The listing builds one solid part. Answer for the finished solid, in the listing's coordinates (mm). A direction names the side the tool comes from. Give positions to 0.01 mm unless a question says otherwise; leave off trailing zeros. Loops run counter-clockwise (first coordinate to the right, second up) from the corner with the lowest first, then second, coordinate; pieces in that order, holes last. Notation, with made-up numbers: M 44,25.25 L 61,25.25 A17 ccw 61,36.25 Z; hole C -39,60.25 d4. An arc over 180 degrees is marked long. Use one line per item in the form item = value. Start each with the question number.
1. The part is cut by section A-A (z = -1). Write down the section's boundary in (x, y).
2. The part is cut by section C-C (y = 14). Write down the section's boundary in (x, z), and give its area (3 significant figures).
3. Each of these flat-tipped pins is pushed along its axis until it touches: pin 1 Ø12 at (y, z) = (31.5, 9) entering from +X; pin 2 Ø19 at (x, z) = (2, -1) entering from +Y. Where does it stop, or does it pass through?
4. The part is cut by section B-B (x = -1.5). Write down the section's boundary in (y, z), and give its area (3 significant figures).
5. Straight lines are drawn through the part: line 1 (X direction, y = 32, z = -8.5); line 2 (Y direction, x = -4, z = 17). For each, find the intervals that lie inside material, in ascending order. Write a range as from..to.
6. For faces 1 (the face through (-25, 40, 0)), 2 (the face through (-23.75, 21, 0)), determine the directions among +Z, -Z, +X, -X, +Y, -Y from which every point of the face is accessible in a straight line to the end or side of a thin tool.
from build123d import *

# Parameters (mm, degrees)
SKETCH1_W           = 51.5
SKETCH1_H           = 37.5
BOSS_EXTRUDE1_DEPTH = 40
SKETCH2_W           = 49.5
SKETCH2_H           = 38
CUT_EXTRUDE1_DEPTH  = 38.5
FILLET1_R           = 1
FILLET2_R           = 2


with BuildPart() as part:
    # Sketch1 → Boss-Extrude1 (new body)
    with BuildSketch(Plane(origin=(0, 0, 0), x_dir=(1, 0, 0), z_dir=(0, 1, 0))):
        Rectangle(SKETCH1_W, SKETCH1_H)
    extrude(amount=BOSS_EXTRUDE1_DEPTH)

    # Sketch2 → Cut-Extrude1 (cut, through all)
    with BuildSketch(Plane.XY.offset(18.75)):
        with Locations((1, 21)):
            Rectangle(SKETCH2_W, SKETCH2_H)
    extrude(amount=-CUT_EXTRUDE1_DEPTH, mode=Mode.SUBTRACT)

    # Fillet1
    fillet1_edges = [part.edges().sort_by_distance(p)[0] for p in [
        (-23.75, 2, 0),
    ]]
    fillet(fillet1_edges, radius=FILLET1_R)

    # Fillet2
    fillet2_edges = [part.edges().sort_by_distance(p)[0] for p in [
        (-25.75, 0, 0),
    ]]
    fillet(fillet2_edges, radius=FILLET2_R)


solid = part.part
Derived:
q1.outline = M -25.75,2 A2 ccw -23.75,0 L 25.75,0 L 25.75,2 L -22.75,2 A1 cw -23.75,3 L -23.75,40 L -25.75,40 Z
q2.outline = M -25.75,-18.75 L -23.75,-18.75 L -23.75,18.75 L -25.75,18.75 Z
q2.area = 75.0 mm2
q3.pin_1 = -23.75
q3.pin_2 = 2
q4.outline = M 0,-18.75 L 2,-18.75 L 2,18.75 L 0,18.75 Z
q4.area = 75.0 mm2
q5.line_1 = -25.75..-23.75
q5.line_2 = 0..2
q6.face_1 = +Z, -Z, +X, -X, +Y
q6.face_2 = +Z, -Z, +X, +Y
